The drawing under review shows one solid part. Ordinate dimensions are in mm from its lowest x, y, z. A direction names the side the tool comes from. Round coordinates to 2 decimals unless told otherwise and drop trailing zeros. Order: outer loops, then holes, each group sorted by start corner. A loop starts at its lowest first (then second) coordinate and runs counter-clockwise, first axis right, second up.
1) Consider section B-B (y = 1.25). Give the boundary of the cut face in (x, z), then the cut area to 3 significant figures.
2) Clearance check with flat-ended pins moving along their axes: P1, Ø1.2, axis at x = 7.5, y = 2.5, coming from the +Z side; P2, Ø6, axis at x = 12.5, z = 8.5, coming from the +Y side; P3, Ø1.8, axis at x = 8.5, y = 3, coming from the -Z side. State where each tip first meets the part, or that it passes through.
3) Consider section A-A (z = 14.1). Give the boundary of the cut face in (x, y).
4) Mouldability with a two-part tool opening along Z and no side actions: class the marked faces 3, 4, 5 and 6 as pulls with the +Z half, pulls with the -Z half, needs draft (parallel to the pull), parting line crosses it, or undercut.
5) Consider section D-D (x = 2.5). Give the boundary of the cut face in (y, z).
6) Consider section C-C (z = 2.25). Give the boundary of the cut face in (x, y), then the cut area to 3 significant figures.
7) Machinability: for the marked faces 1 and 2, which of the approach directions +Z, -Z, +X, -X, +Y, -Y give a long, thin tool a straight path to every point of the face, cutting with its end or side? Answer none if there is none.
8) To check wall thickness, follow L1, parallel to X at y = 1.3, z = 14.1; L2, parallel to Y at x = 13.5, z = 6; L3, parallel to X at y = 2, z = 8.25. State the ranges of each line that lie inside material, in increasing order.
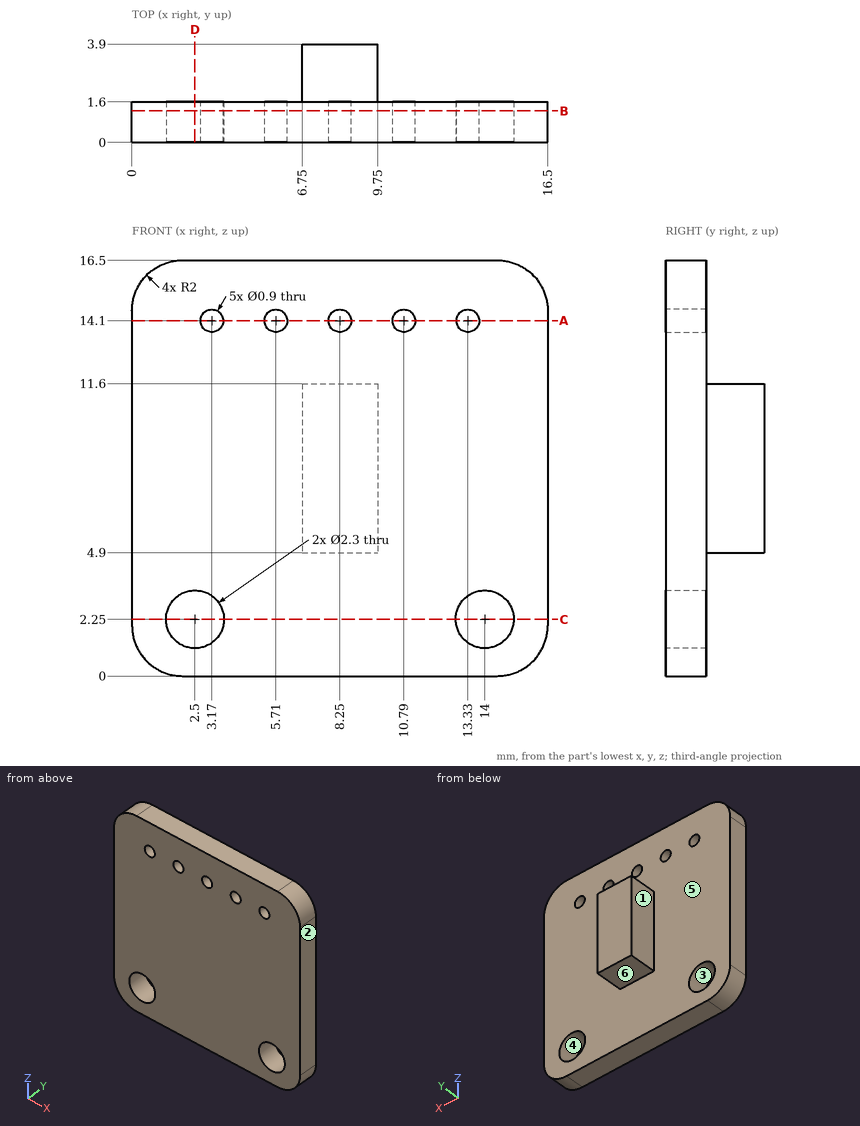
Answer below:
1. outline: (0, 2) arc R2 ccw to (2, 0) - (14.5, 0) arc R2 ccw to (16.5, 2) - (16.5, 14.5) arc R2 ccw to (14.5, 16.5) - (2, 16.5) arc R2 ccw to (0, 14.5) - close; hole circle Ø2.3 at (2.5, 2.25); hole circle Ø0.9 at (3.17, 14.1); hole circle Ø0.9 at (5.71, 14.1); hole circle Ø0.9 at (8.25, 14.1); hole circle Ø0.9 at (10.79, 14.1); hole circle Ø2.3 at (14, 2.25); hole circle Ø0.9 at (13.33, 14.1)
1. area: 257 mm2
2. P1: stops at z = 11.6
2. P2: stops at y = 3.9
2. P3: stops at z = 4.9
3. outline: (0, 0) - (2.72, 0) - (2.72, 1.6) - (0, 1.6) - close; (3.62, 0) - (5.26, 0) - (5.26, 1.6) - (3.62, 1.6) - close; (6.16, 0) - (7.8, 0) - (7.8, 1.6) - (6.16, 1.6) - close; (8.7, 0) - (10.34, 0) - (10.34, 1.6) - (8.7, 1.6) - close; (11.24, 0) - (12.88, 0) - (12.88, 1.6) - (11.24, 1.6) - close; (13.78, 0) - (16.5, 0) - (16.5, 1.6) - (13.78, 1.6) - close
4. face 3: undercut
4. face 4: undercut
4. face 5: needs draft
4. face 6: pulls with the -Z half
5. outline: (0, 0) - (1.6, 0) - (1.6, 1.1) - (0, 1.1) - close; (0, 3.4) - (1.6, 3.4) - (1.6, 16.5) - (0, 16.5) - close
6. outline: (0, 0) - (1.35, 0) - (1.35, 1.6) - (0, 1.6) - close; (3.65, 0) - (12.85, 0) - (12.85, 1.6) - (3.65, 1.6) - close; (15.15, 0) - (16.5, 0) - (16.5, 1.6) - (15.15, 1.6) - close
6. area: 19.0 mm2
7. face 1: +Z, -Z, -X, +Y
7. face 2: +Z, -Z, +X, +Y, -Y
8. L1: x = 0 to 2.72, 3.62 to 5.26, 6.16 to 7.8, 8.7 to 10.34, 11.24 to 12.88, 13.78 to 16.5
8. L2: y = 0 to 1.6
8. L3: x = 6.75 to 9.75
